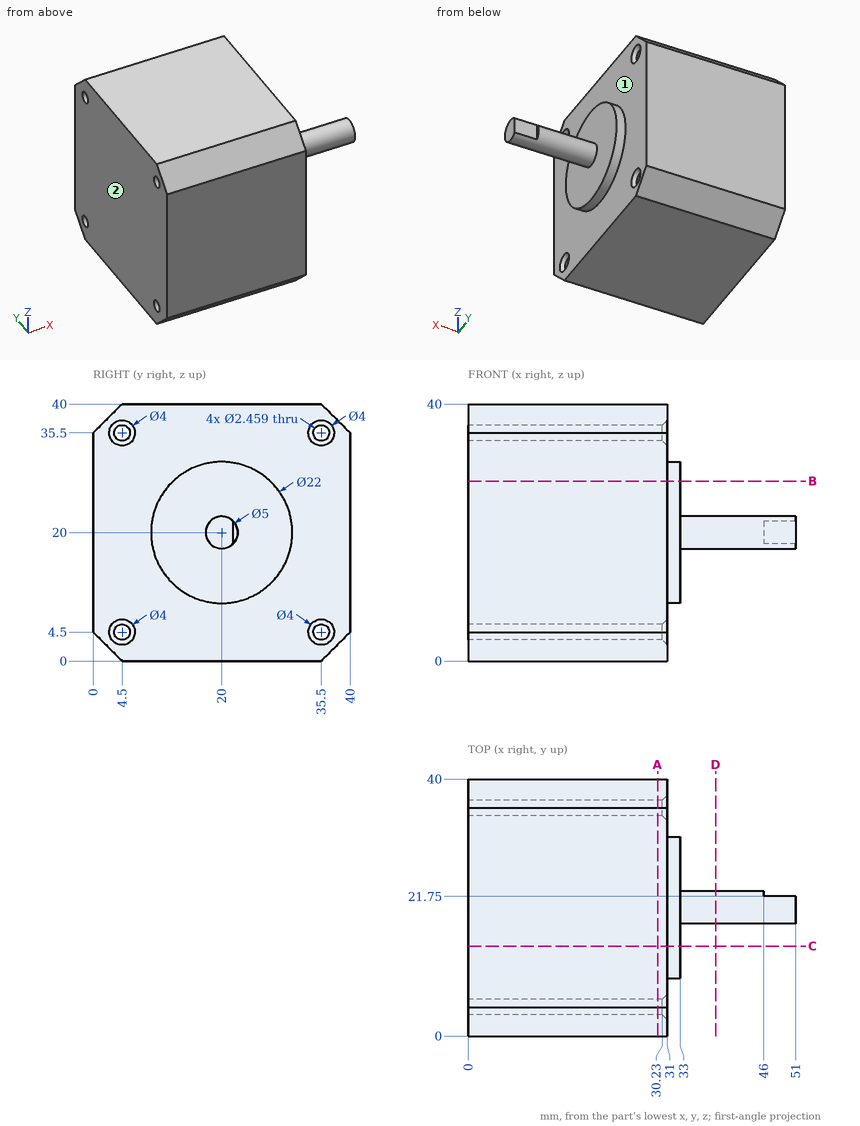
Source: three-view drawing plus pictorial views. Frame: mm from the lowest corner of the part. A direction names the side the tool comes from. Coordinates: 2 decimals unless noted, no trailing zeros. Order: outer loops, then holes, each group sorted by start corner. A loop starts at its lowest first (then second) coordinate and runs counter-clockwise, first axis right, second up. Notation, with made-up numbers: M 25.5,8.5 L 53.5,8.5 A12 ccw 53.5,12.5 Z; hole C 25,-27 d4. An arc over 180 degrees is marked long. Answer in a Markdown table with one row per item.
(1) Section query B-B, the plane z = 28. Output: boundary loops of the cut face in (x, y), plus the area to 3 significant figures.
Numbers:
| item | result |
|---|---|
| outline | M 0,0 L 31,0 L 31,12.45 L 33,12.45 L 33,27.55 L 31,27.55 L 31,40 L 0,40 Z |
| area | 1,270 mm^2 |
(2) Access query for the marked faces 1 and 2. Directions: +Z, -Z, +X, -X, +Y, -Y. A direction counts if a zero-diameter tool reaches every point of the face in a straight line with its end or side. Return the directions, or none.
Numbers:
| item | result |
|---|---|
| face 1 | +X |
| face 2 | +Z, -Z, -X, +Y, -Y |
(3) Contact query for flat-ended pins moving along their axis: pin 1 Ø10 at (y, z) = (13, 13.5) entering from +X; pin 2 Ø1.1 at (x, z) = (49.5, 21) entering from +Y; pin 3 Ø3 at (y, z) = (4.5, 35.5) entering from +X; pin 4 Ø2 at (y, z) = (4.5, 4.5) entering from -X. Output: stop coordinate, or through.
Numbers:
| item | result |
|---|---|
| pin 1 | stops at x = 33 |
| pin 2 | stops at y = 21.75 |
| pin 3 | stops at x = 30.5 |
| pin 4 | passes through |
(4) Section query A-A, the plane x = 29.5. Output: boundary loops of the cut face in (y, z), plus the area to 3 significant figures.
Numbers:
| item | result |
|---|---|
| outline | M 0,4.5 L 4.5,0 L 35.5,0 L 40,4.5 L 40,35.5 L 35.5,40 L 4.5,40 L 0,35.5 Z; hole C 4.5,4.5 d2.46; hole C 4.5,35.5 d2.46; hole C 35.5,4.5 d2.46; hole C 35.5,35.5 d2.46 |
| area | 1,540 mm^2 |
(5) Section query C-C, the plane y = 14. Output: boundary loops of the cut face in (x, z).
Numbers:
| item | result |
|---|---|
| outline | M 0,0 L 31,0 L 31,10.78 L 33,10.78 L 33,29.22 L 31,29.22 L 31,40 L 0,40 Z |
(6) Section query D-D, the plane x = 38.5. Output: boundary loops of the cut face in (y, z).
Numbers:
| item | result |
|---|---|
| outline | C 20,20 d5 |
(7) Material intervals for line 1 (Z direction, x = 24.5, y = 35.5); line 2 (Y direction, x = 7, z = 4) (1 decimal), sorted ascending. Write a range as [from, to].
Numbers:
| item | result |
|---|---|
| line 1 | z = [0, 3.27], [5.73, 34.27], [36.73, 40] |
| line 2 | y = [0.5, 3.4], [5.6, 34.4], [36.6, 39.5] |
